Could you check a few things on this model? Use its own coordinates, in mm. A direction names the side the tool comes from. Give positions to 0.01 mm unless a question says otherwise; leave off trailing zeros. Loops run counter-clockwise (first coordinate to the right, second up) from the corner with the lowest first, then second, coordinate; pieces in that order, holes last. Notation, with made-up numbers: M 58.25,-6 L 100.25,-6 A33 cw 100.25,32 Z; hole C 44,-30.75 d10. An arc over 180 degrees is marked long. Answer in a Markdown table with one row per item. Add a question column.
1. If we section it at A-A on x = -2.6: List the corners of the cut face in (y, z) for me.
2. Which directions (+Z, -Z, +X, -X, +Y, -Y) give clear straight access to the entire face, cutting with the end or side of a thin tool? Please do faces 3 (the flat face through (-1.6, 15, -26)), 4 (the cylindrical face through (-2, -21, -28)).
3. Thinking about a two-plate mould opening in Y: for faces 1 (the flat face through (-1.6, 30, 0)), 2 (the cylindrical face through (0.01, -36.12, 8.02)), which applies, released by +Y, released by -Y, zero draft, split by the parting line, or undercut?
4. I need wall thicknesses on line 1 along Z through (x, y) = (1.15, 4.5); line 2 along Y through (x, z) = (0.95, 10.5); line 3 along Z through (x, y) = (-0.45, 22). Which ranges of each line are inside material? Lowest first, please. Write a range as from..to.
5. I'm going to push flat-ended pins straight in: pin 1 Ø2 at (y, z) = (8, 13) entering from +X; pin 2 Ø2 at (x, z) = (-0.5, -16.5) entering from -Y; pin 3 Ø0.8 at (x, y) = (0, 18) entering from +Z. Where does each tip first touch, or does it pass through?
```python
from build123d import *

# Parameters (mm, degrees)
SKETCH1_R                    = 37
BOSS_EXTRUDE1_DEPTH          = 1.4
SKETCH2_R                    = 1.25
CUT_EXTRUDE1_DEPTH           = 3
CHAMFER1_SIZE                = 0.5
CIRPATTERN1_COUNT            = 6
CHAMFER1_OF_CIRPATTERN1_SIZE = 0.5
CHAMFER2_SIZE                = 0.5
SKETCH3_R                    = 1.25
CUT_EXTRUDE2_DEPTH           = 3
CHAMFER3_SIZE                = 0.5
CIRPATTERN2_COUNT            = 6
CHAMFER3_OF_CIRPATTERN2_SIZE = 0.5
SKETCH4_R                    = 4
CUT_EXTRUDE3_DEPTH           = 2.8
CHAMFER4_SIZE                = 1.25
SKETCH5_R                    = 35
SKETCH5_R_2                  = 4
BOSS_EXTRUDE2_DEPTH          = 2
CUT_EXTRUDE4_START           = -0.5
SKETCH6_R                    = 37
SKETCH6_R_2                  = 35
CUT_EXTRUDE4_DEPTH           = 0.5
CUT_EXTRUDE5_DEPTH           = 3
CHAMFER5_SIZE                = 0.5
CIRPATTERN3_COUNT            = 6
CHAMFER5_OF_CIRPATTERN3_SIZE = 0.5
SKETCH2_2_R                  = 1.25
CUT_EXTRUDE6_DEPTH           = 3
CIRPATTERN4_COUNT            = 6


with BuildPart() as part:
    # Sketch1 → Boss-Extrude1 (new, symmetric)
    with BuildSketch(Plane(origin=(0, 0, 0), x_dir=(0, 0, -1), z_dir=(1, 0, 0))):
        Circle(SKETCH1_R)
    extrude(amount=BOSS_EXTRUDE1_DEPTH, both=True)

    # Sketch2 → Cut-Extrude1 (cut)
    with BuildSketch(Plane(origin=(1.4, 0, 0), x_dir=(0, 0, -1), z_dir=(1, 0, 0))):
        with Locations((0, 30)):
            Circle(SKETCH2_R)
    cut_extrude1 = extrude(amount=-CUT_EXTRUDE1_DEPTH, mode=Mode.SUBTRACT)

    # Chamfer1
    chamfer1_edges = [part.edges().sort_by_distance(p)[0] for p in [
        (1.4, 30, 1.25),
    ]]
    chamfer(chamfer1_edges, length=CHAMFER1_SIZE)

    # CirPattern1: Cut-Extrude1 ×6 about axis
    cirpattern1_axis = Axis((0, 0, 0), (1, 0, 0))
    for i in range(1, CIRPATTERN1_COUNT):
        add(cut_extrude1.rotate(cirpattern1_axis, i * 360 / CIRPATTERN1_COUNT), mode=Mode.SUBTRACT)

    # Chamfer1 of CirPattern1
    chamfer1_of_cirpattern1_edges = [part.edges().sort_by_distance(p)[0] for p in [
        (1.4, 13.917468245, 26.605762114),
        (1.4, -16.082531755, 25.355762114),
        (1.4, -30, -1.25),
        (1.4, -13.917468245, -26.605762114),
        (1.4, 16.082531755, -25.355762114),
    ]]
    chamfer(chamfer1_of_cirpattern1_edges, length=CHAMFER1_OF_CIRPATTERN1_SIZE)

    # Chamfer2
    chamfer2_edges = [part.edges().sort_by_distance(p)[0] for p in [
        (1.4, 0, 37),
    ]]
    chamfer(chamfer2_edges, length=CHAMFER2_SIZE)

    # Sketch3 → Cut-Extrude2 (cut)
    with BuildSketch(Plane(origin=(1.4, 0, 0), x_dir=(0, 0, -1), z_dir=(1, 0, 0))):
        with Locations((0, 15)):
            Circle(SKETCH3_R)
    cut_extrude2 = extrude(amount=-CUT_EXTRUDE2_DEPTH, mode=Mode.SUBTRACT)

    # Chamfer3
    chamfer3_edges = [part.edges().sort_by_distance(p)[0] for p in [
        (1.4, 15, 1.25),
    ]]
    chamfer(chamfer3_edges, length=CHAMFER3_SIZE)

    # CirPattern2: Cut-Extrude2 ×6 about axis
    cirpattern2_axis = Axis((0, 0, 0), (1, 0, 0))
    for i in range(1, CIRPATTERN2_COUNT):
        add(cut_extrude2.rotate(cirpattern2_axis, i * 360 / CIRPATTERN2_COUNT), mode=Mode.SUBTRACT)

    # Chamfer3 of CirPattern2
    chamfer3_of_cirpattern2_edges = [part.edges().sort_by_distance(p)[0] for p in [
        (1.4, 6.417468245, 13.615381057),
        (1.4, -8.582531755, 12.365381057),
        (1.4, -15, -1.25),
        (1.4, -6.417468245, -13.615381057),
        (1.4, 8.582531755, -12.365381057),
    ]]
    chamfer(chamfer3_of_cirpattern2_edges, length=CHAMFER3_OF_CIRPATTERN2_SIZE)

    # Sketch4 → Cut-Extrude3 (cut)
    with BuildSketch(Plane(origin=(1.4, 0, 0), x_dir=(0, 0, -1), z_dir=(1, 0, 0))):
        Circle(SKETCH4_R)
    extrude(amount=-CUT_EXTRUDE3_DEPTH, mode=Mode.SUBTRACT)

    # Chamfer4
    chamfer4_edges = [part.edges().sort_by_distance(p)[0] for p in [
        (1.4, 0, 4),
    ]]
    chamfer(chamfer4_edges, length=CHAMFER4_SIZE)

    # Sketch5 → Boss-Extrude2 (add)
    with BuildSketch(Plane.ZY.offset(1.4)):
        Circle(SKETCH5_R)
        with Locations(Location((0, 0, 0), (0, 0, 180))):
            Circle(SKETCH5_R_2, mode=Mode.SUBTRACT)
    extrude(amount=BOSS_EXTRUDE2_DEPTH)

    # Sketch6 → Cut-Extrude4 (cut)
    with BuildSketch(Plane.ZY.offset(1.4).offset(CUT_EXTRUDE4_START)):
        Circle(SKETCH6_R)
        Circle(SKETCH6_R_2, mode=Mode.SUBTRACT)
    extrude(amount=CUT_EXTRUDE4_DEPTH, mode=Mode.SUBTRACT)

    # Sketch7 → Cut-Extrude5 (cut)
    with BuildSketch(Plane(origin=(1.4, 0, 0), x_dir=(0, 0, -1), z_dir=(1, 0, 0))):
        with BuildLine():
            Line((-5.150629559, 13.185920405), (-5.150629559, 28.104599213))
            ThreePointArc((-5.150629559, 28.104599213), (-5.923090095, 29.683569404), (-7.643776425, 30.042847434))
            ThreePointArc((-7.643776425, 30.042847434), (-15.5, 26.846787517), (-22.195980868, 21.641128282))
            ThreePointArc((-22.195980868, 21.641128282), (-22.745180132, 19.971331194), (-21.763982102, 18.51287565))
            Line((-21.763982102, 18.51287565), (-8.844027263, 11.053536246))
            ThreePointArc((-8.844027263, 11.053536246), (-7.817335996, 10.785765167), (-6.798156961, 11.080842113))
            ThreePointArc((-6.798156961, 11.080842113), (-6.5, 11.258330249), (-6.197212284, 11.427797684))
            ThreePointArc((-6.197212284, 11.427797684), (-5.432078636, 12.162894146), (-5.150629559, 13.185920405))
        make_face()
    cut_extrude5 = extrude(amount=-CUT_EXTRUDE5_DEPTH, mode=Mode.SUBTRACT)

    # Chamfer5
    chamfer5_edges = [part.edges().sort_by_distance(p)[0] for p in [
        (1.4, 29.683569404, 5.923090095),
        (1.4, 26.846787517, 15.5),
        (1.4, 19.971331194, 22.745180132),
        (1.4, 14.783205948, 15.304004683),
        (1.4, 10.785765167, 7.817335996),
        (1.4, 11.258330249, 6.5),
        (1.4, 12.162894146, 5.432078636),
        (1.4, 20.645259809, 5.150629559),
    ]]
    chamfer(chamfer5_edges, length=CHAMFER5_SIZE)

    # CirPattern3: Cut-Extrude5 ×6 about axis
    cirpattern3_axis = Axis((0, 0, 0), (1, 0, 0))
    for i in range(1, CIRPATTERN3_COUNT):
        add(cut_extrude5.rotate(cirpattern3_axis, i * 360 / CIRPATTERN3_COUNT), mode=Mode.SUBTRACT)

    # Chamfer5 of CirPattern3
    chamfer5_of_cirpattern3_edges = [part.edges().sort_by_distance(p)[0] for p in [
        (1.4, 9.712238211, 28.668270227),
        (1.4, 0, 31),
        (1.4, -9.712238211, 28.668270227),
        (1.4, -5.862053861, 20.454634241),
        (1.4, -1.377128979, 13.249414632),
        (1.4, 0, 13),
        (1.4, 1.377128979, 13.249414632),
        (1.4, 5.862053861, 20.454634241),
        (1.4, -19.971331194, 22.745180132),
        (1.4, -26.846787517, 15.5),
        (1.4, -29.683569405, 5.923090095),
        (1.4, -20.645259809, 5.150629559),
        (1.4, -12.162894146, 5.432078636),
        (1.4, -11.258330249, 6.5),
        (1.4, -10.785765167, 7.817335996),
        (1.4, -14.783205948, 15.304004683),
        (1.4, -29.683569404, -5.923090095),
        (1.4, -26.846787517, -15.5),
        (1.4, -19.971331194, -22.745180132),
        (1.4, -14.783205948, -15.304004683),
        (1.4, -10.785765167, -7.817335996),
        (1.4, -11.258330249, -6.5),
        (1.4, -12.162894146, -5.432078636),
        (1.4, -20.645259809, -5.150629559),
        (1.4, -9.712238211, -28.668270227),
        (1.4, 0, -31),
        (1.4, 9.712238211, -28.668270227),
        (1.4, 5.862053861, -20.454634241),
        (1.4, 1.377128979, -13.249414632),
        (1.4, 0, -13),
        (1.4, -1.377128979, -13.249414632),
        (1.4, -5.862053861, -20.454634241),
        (1.4, 19.971331194, -22.745180132),
        (1.4, 26.846787517, -15.5),
        (1.4, 29.683569405, -5.923090095),
        (1.4, 20.645259809, -5.150629559),
        (1.4, 12.162894146, -5.432078636),
        (1.4, 11.258330249, -6.5),
        (1.4, 10.785765167, -7.817335996),
        (1.4, 14.783205948, -15.304004683),
    ]]
    chamfer(chamfer5_of_cirpattern3_edges, length=CHAMFER5_OF_CIRPATTERN3_SIZE)

    # Sketch2<2> → Cut-Extrude6 (cut)
    with BuildSketch(Plane(origin=(1.4, 0, 0), x_dir=(0, 0, -1), z_dir=(1, 0, 0))):
        with Locations((0, 30)):
            Circle(SKETCH2_2_R)
    cut_extrude6 = extrude(amount=-CUT_EXTRUDE6_DEPTH, mode=Mode.SUBTRACT)

    # CirPattern4: Cut-Extrude6 ×6 about axis
    cirpattern4_axis = Axis((1.4, 0, 0), (-1, 0, 0))
    for i in range(1, CIRPATTERN4_COUNT):
        add(cut_extrude6.rotate(cirpattern4_axis, i * 360 / CIRPATTERN4_COUNT), mode=Mode.SUBTRACT)


solid = part.part
```
Results:
| question | item | result |
|---|---|---|
| 1 | outline | C 0,0 d70; hole C 0,0 d8 |
| 2 | face 3 | +X |
| 2 | face 4 | -X |
| 3 | face 1 | undercut |
| 3 | face 2 | split by the parting line |
| 4 | line 1 | -36.47..-30.92, -17.6..-2.18, 2.18..17.6, 30.92..36.47 |
| 4 | line 2 | -35.43..-29.22, -11.95..11.95, 29.22..35.43 |
| 4 | line 3 | -29.75..-21.84, -5.15..5.15, 21.84..29.75 |
| 5 | pin 1 | x = 1.15 |
| 5 | pin 2 | y = -33.6 |
| 5 | pin 3 | z = 32.55 |
